Geometry check sheet. Reference: the model listing, model coordinates, mm. Face numbers are marked on the shaded views. A direction names the side the tool comes from. Coordinates: 2 decimals unless noted, no trailing zeros. Order: outer loops, then holes, each group sorted by start corner. A loop starts at its lowest first (then second) coordinate and runs counter-clockwise, first axis right, second up. Notation, with made-up numbers: M 28.5,42 L 46.5,42 A19 ccw 46.5,76 Z; hole C 42.25,82 d3. An arc over 180 degrees is marked long. One line per item, written item: value. Start each with the question number.
1) Sectioned sample at A-A, the plane x = 0. Enter the section's corners in (y, z).
2) Sectioned sample at B-B, the plane z = -2.5. Enter the section's corners in (x, y), then the cut area to 3 significant figures.
3) Go/stop test with flat-tipped pins: P1, Ø15, axis at x = -9.5, y = 11.5, coming from the -Z side; P2, Ø8, axis at x = -10, y = 25.5, coming from the +Z side; P3, Ø3, axis at y = 23.5, z = -9.5, coming from the -X side. Record where each tip stops, or that it passes through.
4) Sectioned sample at D-D, the plane z = -9.5. Enter the section's corners in (x, y), then the cut area to 3 significant figures.
5) Sectioned sample at C-C, the plane y = 24.5. Enter the section's corners in (x, z), then the cut area to 3 significant figures.
6) Access from +Z, -Z, +X, -X, +Y, -Y to the whole of each face (thin tool, end or side, straight path). Record for the marked faces 4, 5, 6, 7 and 8.
7) Draft check along Z on the marked faces 1, 2 and 3. Enter one of: pulls with the +Z half, pulls with the -Z half, needs draft (parallel to the pull), parting line crosses it, or undercut.
8) Thickness scan on L1, parallel to Z at x = -2.5, y = 8.75; L2, parallel to Y at x = 0, z = -12; L3, parallel to Y at x = -15.5, z = -8. Record the ranges inside material, lowest first. Write a range as from..to.
```python
from build123d import *

# Parameters (mm, degrees)
SKETCH1_W           = 40.5
SKETCH1_H           = 30.5
SKETCH1_W_2         = 20.5
SKETCH1_H_2         = 10.5
BOSS_EXTRUDE1_DEPTH = 19.5
SKETCH4_R           = 1
BOSS_EXTRUDE2_DEPTH = 3
SKETCH3_W           = 18.5
SKETCH3_H           = 10
SKETCH3_R           = 2.25
BOSS_EXTRUDE3_DEPTH = 10


with BuildPart() as part:
    # Sketch1 → Boss-Extrude1 (new body)
    with BuildSketch(Plane(origin=(0, 0, 0), x_dir=(1, 0, 0), z_dir=(0, 1, 0))):
        Rectangle(SKETCH1_W, SKETCH1_H)
        Rectangle(SKETCH1_W_2, SKETCH1_H_2, mode=Mode.SUBTRACT)
    extrude(amount=BOSS_EXTRUDE1_DEPTH)

    # Sketch4 → Boss-Extrude2 (add)
    with BuildSketch(Plane.XY.offset(-15.25)):
        with Locations((0, 4.5)):
            Circle(SKETCH4_R)
    extrude(amount=-BOSS_EXTRUDE2_DEPTH)

    # Sketch3 → Boss-Extrude3 (add)
    with BuildSketch(Plane(origin=(0, 0, -15.25), x_dir=(-1, 0, 0), z_dir=(0, 0, -1))):
        with Locations((0, 24.5)):
            Rectangle(SKETCH3_W, SKETCH3_H)
        with Locations((0, 24.5)):
            Circle(SKETCH3_R, mode=Mode.SUBTRACT)
    extrude(amount=-BOSS_EXTRUDE3_DEPTH)


solid = part.part
```
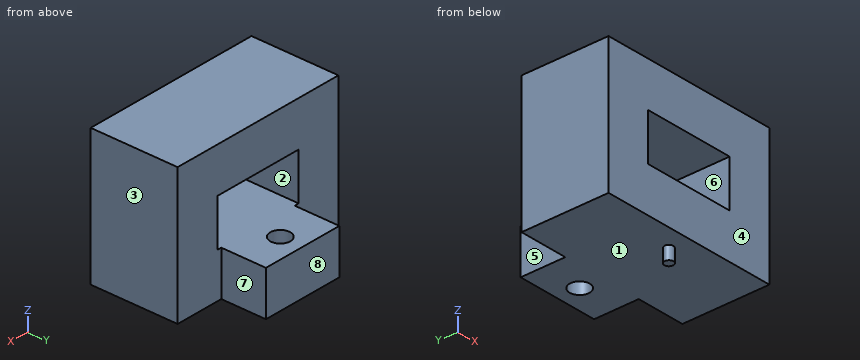
Final values:
1. outline: M 0,-15.25 L 3.5,-15.25 L 3.5,-18.25 L 5.5,-18.25 L 5.5,-15.25 L 22.25,-15.25 L 22.25,-5.25 L 0,-5.25 Z; M 0,5.25 L 19.5,5.25 L 19.5,15.25 L 0,15.25 Z; M 26.75,-15.25 L 29.5,-15.25 L 29.5,-5.25 L 26.75,-5.25 Z
2. outline: M -20.25,0 L -10.25,0 L -10.25,19.5 L -20.25,19.5 Z; M 10.25,0 L 20.25,0 L 20.25,19.5 L 10.25,19.5 Z
2. area: 390 mm^2
3. P1: stops at z = -15.25
3. P2: stops at z = -5.25
3. P3: stops at x = -9.25
4. outline: M -20.25,0 L 20.25,0 L 20.25,19.5 L 9.25,19.5 L 9.25,29.5 L -9.25,29.5 L -9.25,19.5 L -20.25,19.5 Z; hole C 0,24.5 d4.5
4. area: 959 mm^2
5. outline: M -9.25,-15.25 L -2.25,-15.25 L -2.25,-5.25 L -9.25,-5.25 Z; M 2.25,-15.25 L 9.25,-15.25 L 9.25,-5.25 L 2.25,-5.25 Z
5. area: 140 mm^2
6. face 4: +Z, -Z, +X, -X, -Y
6. face 5: +Z, -Z, -X, +Y
6. face 6: +Y, -Y
6. face 7: +Z, -Z, +X, +Y
6. face 8: +Z, -Z, +X, -X, +Y
7. face 1: pulls with the -Z half
7. face 2: undercut
7. face 3: needs draft
8. L1: z = -15.25..-5.25, 5.25..15.25
8. L2: y = 0..22.25, 26.75..29.5
8. L3: y = 0..19.5
